```python
from build123d import *

# Parameters (mm, degrees)
SKETCH2_R          = 6.477
CUT_EXTRUDE1_DEPTH = 37.411588815
CHAMFER1_SIZE      = 1.27


with BuildPart() as part:
    # Sketch1 → Revolve1 (revolve)
    with BuildSketch(Plane(origin=(0, 0, 0), x_dir=(0, 0, -1), z_dir=(1, 0, 0))):
        with BuildLine():
            Line((0, 0), (24.13, 0))
            Line((24.13, 0), (24.13, 2.54))
            ThreePointArc((24.13, 2.54), (20.32, 6.35), (24.13, 10.16))
            Line((24.13, 10.16), (24.13, 12.7))
            Line((24.13, 12.7), (0, 12.7))
            Line((0, 12.7), (0, 0))
        make_face()
    revolve(axis=Axis((0, 0, 0), (0, 1, 0)))

    # Sketch2 → Cut-Extrude1 (cut, through all)
    with BuildSketch(Plane.XZ):
        with Locations(Location((0, 0, 0), (0, 0, 270))):
            Circle(SKETCH2_R)
    extrude(amount=-CUT_EXTRUDE1_DEPTH, mode=Mode.SUBTRACT)

    # Chamfer1
    chamfer1_edges = [part.edges().sort_by_distance(p)[0] for p in [
        (0, 12.7, 6.477),
        (0, 0, 6.477),
    ]]
    chamfer(chamfer1_edges, length=CHAMFER1_SIZE)


solid = part.part
```
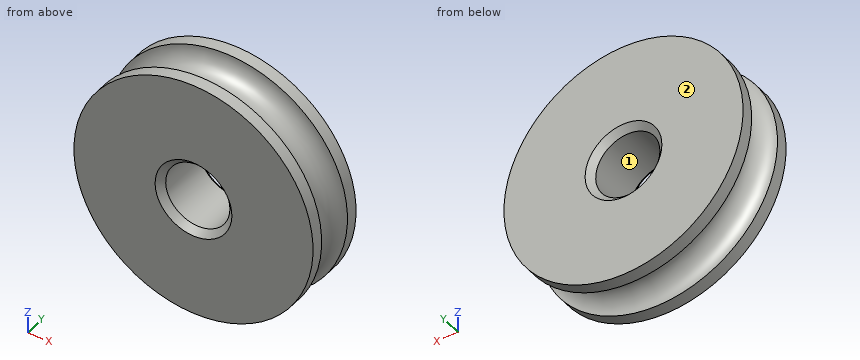
Can you work these out from the model? Positions are in its coordinate system, mm. Face numbers are marked on the shaded views. Give positions to 0.01 mm unless a question says otherwise; leave off trailing zeros. Order: outer loops, then holes, each group sorted by start corner. A loop starts at its lowest first (then second) coordinate and runs counter-clockwise, first axis right, second up. Notation, with made-up numbers: M 80.25,32.5 L 117.25,32.5 A19 cw 117.25,51.5 Z; hole C -11,-6.5 d7. An arc over 180 degrees is marked long. Write item = value, one per line. Start each with the question number.
Q1. Will these pins go through, and if not, where does the flat tip stop? pin 1 Ø6 at (y, z) = (3.5, 0) entering from +X; pin 2 Ø3 at (x, y) = (-16, 2) entering from +Z; pin 3 Ø4 at (y, z) = (7, -13.5) entering from +X.
Q2. I need wall thicknesses on probe 1 along Y at (x, z) = (21, -6); probe 2 along X at (y, z) = (5, 0); probe 3 along X at (y, z) = (6.25, 0). Which ranges of each line are inside material? Lowest first, please. Write a range as [from, to].
Q3. Suppose I cut it at B-B (x = 0). Write out the boundary of the cut face in (y, z), plus the area to 3 significant figures.
Q4. Suppose I cut it at D-D (y = 6.25). Write out the boundary of the cut face in (x, z), plus the area to 3 significant figures.
Q5. We'd pull the mould along Z, two halves only. Please class the marked faces 1 and 2: pulls with the +Z half, pulls with the -Z half, needs draft (parallel to the pull), parting line crosses it, or undercut.
Q6. Suppose I cut it at C-C (y = 10.75). Write out the boundary of the cut face in (x, z).
Q7. Suppose I cut it at A-A (z = 0). Write out the boundary of the cut face in (x, y).
Check result:
q1.pin_1 = 24.13
q1.pin_2 = 19.29
q1.pin_3 = 17.09
q2.probe_1 = [0, 3.3], [9.4, 12.7]
q2.probe_2 = [-20.57, -6.48], [6.48, 20.57]
q2.probe_3 = [-20.32, -6.48], [6.48, 20.32]
q3.outline = M 0,-24.13 L 2.54,-24.13 A3.81 cw 10.16,-24.13 L 12.7,-24.13 L 12.7,-7.75 L 11.43,-6.48 L 1.27,-6.48 L 0,-7.75 Z; M 0,7.75 L 1.27,6.48 L 11.43,6.48 L 12.7,7.75 L 12.7,24.13 L 10.16,24.13 A3.81 cw 2.54,24.13 L 0,24.13 Z
q3.area = 400 mm2
q4.outline = C 0,0 d40.64; hole C 0,0 d12.95
q4.area = 1,170 mm2
q5.face_1 = undercut
q5.face_2 = needs draft
q6.outline = C 0,0 d48.26; hole C 0,0 d12.95
q7.outline = M -24.13,0 L -7.75,0 L -6.48,1.27 L -6.48,11.43 L -7.75,12.7 L -24.13,12.7 L -24.13,10.16 A3.81 cw -24.13,2.54 Z; M 6.48,1.27 L 7.75,0 L 24.13,0 L 24.13,2.54 A3.81 cw 24.13,10.16 L 24.13,12.7 L 7.75,12.7 L 6.48,11.43 Z
